from build123d import *

# Parameters (mm, degrees)
F0_W     = 80
F0_H     = 50
F1_DEPTH = 10
F2_T     = -2
F3_R     = 1.5
F4_DEPTH = 25


with BuildPart() as f1:
    # F0 (on Top) → F1 (new body)
    with BuildSketch(Plane.XY):
        Rectangle(F0_W, F0_H)
    extrude(amount=F1_DEPTH)

    # F2
    f2_openings = [f1.faces().sort_by_distance(p)[0] for p in [
        (0, 0, 10),
        (0, 0, 0),
    ]]
    offset(amount=F2_T, openings=f2_openings)

    # F3 (on Front) → F4 (cut, symmetric)
    with BuildSketch(Plane.XZ):
        with Locations((0, 5)):
            Circle(F3_R)
        with Locations((30, 5)):
            Circle(F3_R)
        with Locations((-30, 5)):
            Circle(F3_R)
    extrude(amount=F4_DEPTH, both=True, mode=Mode.SUBTRACT)


solid = f1.part
Can you work these out from the model? Positions are in its coordinate system, mm. A direction names the side the tool comes from. Give positions to 0.01 mm unless a question says otherwise; leave off trailing zeros. Loops run counter-clockwise (first coordinate to the right, second up) from the corner with the lowest first, then second, coordinate; pieces in that order, holes last. Notation, with made-up numbers: (56, -31) - (83, -31) arc R4 cw to (83, -25) - close; hole circle Ø11 at (44, 36). An arc over 180 degrees is marked (long way). Answer as a JSON object with one key per item and string values.
Q1. Will this pin go through, and if not, where does the flat tip stop? P1, Ø3.5, axis at x = -30, z = 5, coming from the +Y side.
Geometry says:
{"P1": "y = 25"}
Q2. Imagine slicing it at D-D on x = -6. Write out the boundary of the cut face in (y, z).
Geometry says:
{"outline": "(-25, 0) - (-23, 0) - (-23, 10) - (-25, 10) - close; (23, 0) - (25, 0) - (25, 10) - (23, 10) - close"}
Q3. Imagine slicing it at C-C on y = -11. Write out the boundary of the cut face in (x, z).
Geometry says:
{"outline": "(-40, 0) - (-38, 0) - (-38, 10) - (-40, 10) - close; (38, 0) - (40, 0) - (40, 10) - (38, 10) - close"}
Q4. If we mould it in two halves opening along Z, with no side actions, what happens to faces 1 (the flat face through (-1, -25, 3)), 2 (the cylindrical face through (-1.5, 23.99, 5.07)), 3 (the flat face through (-3, -24, 10))? For each: pulls with the +Z half, pulls with the -Z half, needs draft (parallel to the pull), parting line crosses it, or undercut.
Geometry says:
{"face 1": "needs draft", "face 2": "undercut", "face 3": "pulls with the +Z half"}
Q5. Imagine slicing it at B-B on x = -30. Write out the boundary of the cut face in (y, z).
Geometry says:
{"outline": "(-25, 0) - (-23, 0) - (-23, 3.5) - (-25, 3.5) - close; (-25, 6.5) - (-23, 6.5) - (-23, 10) - (-25, 10) - close; (23, 0) - (25, 0) - (25, 3.5) - (23, 3.5) - close; (23, 6.5) - (25, 6.5) - (25, 10) - (23, 10) - close"}
Q6. Imagine slicing it at A-A on z = 5. Give the number of separate pieces and of enclosed holes in the cut face, plus the area to 3 significant figures.
Geometry says:
{"separate pieces": "6", "enclosed holes": "0", "area": "468 mm²"}
Q7. If I drill on L1, parallel to Y at x = 35, z = 8; L2, parallel to X at y = -18, z = 3.75; L3, parallel to Z at x = 0, y = -24, over which ranges is the centre line in solid material (lowest first)?
Geometry says:
{"L1": "-25 to -23, 23 to 25", "L2": "-40 to -38, 38 to 40", "L3": "0 to 3.5, 6.5 to 10"}
Q8. Which directions (+Z, -Z, +X, -X, +Y, -Y) give clear straight access to the entire face, cutting with the end or side of a thin tool? Please do faces 4 (the flat face through (-3, -24, 0)), 5 (the flat face through (-38, 0, 5)).
Geometry says:
{"face 4": "-Z, +X, -X, +Y, -Y", "face 5": "+Z, -Z"}
